from build123d import *

# Parameters (mm, degrees)
SKETCH1_W           = 55
SKETCH1_H           = 80
BOSS_EXTRUDE1_DEPTH = 3
SKETCH2_R           = 2.185
SKETCH2_R_2         = 1.984375
CUT_EXTRUDE1_DEPTH  = 4
CUT_EXTRUDE2_DEPTH  = 4
FILLET1_R           = 10


with BuildPart() as part:
    # Sketch1 → Boss-Extrude1 (new body)
    with BuildSketch(Plane(origin=(0, 0, 0), x_dir=(1, 0, 0), z_dir=(0, 1, 0))):
        Rectangle(SKETCH1_W, SKETCH1_H)
    extrude(amount=BOSS_EXTRUDE1_DEPTH)

    # Sketch2 → Cut-Extrude1 (cut, through all)
    with BuildSketch(Plane(origin=(0, 3, 0), x_dir=(1, 0, 0), z_dir=(0, 1, 0))):
        with Locations((0, 8.25)):
            Circle(SKETCH2_R)
        with Locations((0, -23.271)):
            Circle(SKETCH2_R)
        with Locations((-19.5625, 27)):
            Circle(SKETCH2_R_2)
        with Locations((-19.5625, 1.6)):
            Circle(SKETCH2_R_2)
        with Locations((19.5625, 27)):
            Circle(SKETCH2_R_2)
        with Locations((19.5625, 1.6)):
            Circle(SKETCH2_R_2)
    extrude(amount=-CUT_EXTRUDE1_DEPTH, mode=Mode.SUBTRACT)

    # Sketch3 → Cut-Extrude2 (cut, through all)
    with BuildSketch(Plane(origin=(0, 3, 0), x_dir=(1, 0, 0), z_dir=(0, 1, 0))):
        Polygon((18.510308796, -29.09449619), (0, -40), (27.5, -40), (27.5, 10.752872816), align=None)
    cut_extrude2 = extrude(amount=-CUT_EXTRUDE2_DEPTH, mode=Mode.SUBTRACT)

    # Mirror1: Cut-Extrude2 across plane
    add(cut_extrude2.mirror(Plane(origin=(0, 0, 0), x_dir=(0, 0, 1), z_dir=(1, 0, 0))), mode=Mode.SUBTRACT)

    # Fillet1
    fillet1_edges = [part.edges().sort_by_distance(p)[0] for p in [
        (18.510308796, 1.5, 29.09449619),
        (0, 1.5, 40),
        (-18.510308796, 1.5, 29.09449619),
    ]]
    fillet(fillet1_edges, radius=FILLET1_R)


solid = part.part
Design review of the part built by this model. Coordinates are the model's own, in mm. Round coordinates to 2 decimals unless told otherwise and drop trailing zeros. Write each loop counter-clockwise with the first axis right and the second up, starting at its lowest first coordinate (ties: lowest second). Pieces come first, ordered by that corner, then holes.
Item 1: Consider section A-A on z = -27. Give the boundary of the cut face in (x, y), and give its area (3 significant figures).
Item 2: Draft analysis for pull direction Z (two halves, no side actions). For faces 1 (the cylindrical face through (0.075, 1.479, 38.393)), 2 (the cylindrical face through (-21.545, 1.521, -1.687)), 3 (the flat face through (-27.5, 1, -25)), state which applies: released by +Z, released by -Z, zero draft, split by the parting line, or undercut.
Item 3: Consider section B-B on x = 0. Give the boundary of the cut face in (y, z) (1 decimal).
Item 4: For pin 1 Ø1 at (y, z) = (1.5, 13.5) entering from +X; pin 2 Ø1.5 at (y, z) = (2.5, 7) entering from +X, all flat-tipped, find the tip position at first contact; note any pin that passes through.
Item 5: Wall thickness on L1, parallel to X at y = 2.05, z = -27; L2, parallel to Z at x = -18, y = 0.8; L3, parallel to X at y = 2.15, z = -1.6: over which ranges is each line inside the solid? List them lowest first.
Item 6: Consider section D-D on y = 0.95. Count the separate pieces of the cut face and the enclosed holes in it, and give its area (3 significant figures).
Item 7: Consider section C-C on z = -8.25. Give the boundary of the cut face in (x, y) (3 decimals), and give its area (3 significant figures).
Check values:
1. outline: (-27.5, 0) - (-21.55, 0) - (-21.55, 3) - (-27.5, 3) - close; (-17.58, 0) - (17.58, 0) - (17.58, 3) - (-17.58, 3) - close; (21.55, 0) - (27.5, 0) - (27.5, 3) - (21.55, 3) - close
1. area: 141 mm2
2. face 1: released by +Z
2. face 2: undercut
2. face 3: zero draft
3. outline: (0, -40) - (3, -40) - (3, -10.4) - (0, -10.4) - close; (0, -6.1) - (3, -6.1) - (3, 21.1) - (0, 21.1) - close; (0, 25.5) - (3, 25.5) - (3, 38.4) - (0, 38.4) - close
4. pin 1: stops at x = 22.14
4. pin 2: stops at x = 23.66
5. L1: x = -27.5 to -21.55, -17.58 to 17.58, 21.55 to 27.5
5. L2: z = -40 to -28.22, -25.78 to -2.82, -0.38 to 28.26
5. L3: x = -25.44 to -21.55, -17.58 to 17.58, 21.55 to 25.44
6. separate pieces: 1
6. enclosed holes: 6
6. area: 3,550 mm2
7. outline: (-26.935, 0) - (-2.185, 0) - (-2.185, 3) - (-26.935, 3) - close; (2.185, 0) - (26.935, 0) - (26.935, 3) - (2.185, 3) - close
7. area: 149 mm2
